Build history of the part. All positions in model axes, mm. Round coordinates to 2 decimals unless told otherwise and drop trailing zeros. Answer in a Markdown table with one row per item.
```python
from build123d import *

# Parameters (mm, degrees)
F1_DEPTH = 3.96875
F2_D     = 6.35
F3_D     = 6.35


with BuildPart() as f1:
    # F0 (on Top) → F1 (new body)
    with BuildSketch(Plane.XY):
        with BuildLine():
            add(Edge.make_bspline(
                [(93.0961013775, 11.8631264067), (73.0208323512, -1.8265877953), (59.8314115865, 0), (7.6732839915, 0)],
                knots=[0, 0, 0, 0, 86.2426315595, 86.2426315595, 86.2426315595, 86.2426315595], degree=3))
            add(Edge.make_bspline(
                [(7.3635370912, 22.8609638917), (45.8569088961, 23.6332072416), (80.4890639518, 17.6334698365), (93.0961013775, 11.8631264067)],
                knots=[0, 0, 0, 0, 86.4350913023, 86.4350913023, 86.4350913023, 86.4350913023], degree=3))
            add(Edge.make_bspline(
                [(-50.7329378175, 20.9600568183), (-28.6348905119, 23.0391732855), (-2.4380154521, 23.6332072416), (7.3635370912, 22.8609638917)],
                knots=[0, 0, 0, 0, 58.1275652726, 58.1275652726, 58.1275652726, 58.1275652726], degree=3))
            add(Edge.make_bspline(
                [(-81.150870805, 19.8313930948), (-72.6527741432, 19.950199886), (-60.8315071405, 19.059149745), (-50.7329378175, 20.9600568183)],
                knots=[0, 0, 0, 0, 30.4388654361, 30.4388654361, 30.4388654361, 30.4388654361], degree=3))
            add(Edge.make_bspline(
                [(-81.150870805, -3.0372931352), (-91.1866208845, 0), (-96.1764965988, 16.4454019242), (-81.150870805, 19.8313930948)],
                knots=[0, 0, 0, 0, 22.8686862301, 22.8686862301, 22.8686862301, 22.8686862301], degree=3))
            add(Edge.make_bspline(
                [(-41.2958105253, -1.8235209079), (-58.2979012822, -1.90700734), (-70.3425093809, 3.5678162715), (-81.150870805, -3.0372931352)],
                knots=[0, 0, 0, 0, 39.8735385051, 39.8735385051, 39.8735385051, 39.8735385051], degree=3))
            add(Edge.make_bspline(
                [(-0.9071079771, -2.6666779982), (-11.7089183609, 7.7004259843), (-20.3979939932, -2.0482919491), (-41.2958105253, -1.8235209079)],
                knots=[0, 0, 0, 0, 40.3975024897, 40.3975024897, 40.3975024897, 40.3975024897], degree=3))
            ThreePointArc((-0.9071079771, -2.6666779982), (2.8162542913, 0.4905240496), (7.6732839915, 0))
        make_face()
    extrude(amount=F1_DEPTH)

    # F2 (through all)
    with Locations(Plane(origin=(0, 0, 0), x_dir=(1, 0, 0), z_dir=(0, 0, -1))):
        with Locations((-49.7787126682, -11.3269922778)):
            Hole(F2_D / 2)

    # F3 (through all)
    with Locations(Plane(origin=(0, 0, 0), x_dir=(1, 0, 0), z_dir=(0, 0, -1))):
        with Locations((-83.2072975638, -10.5645472046), (-17.3172454044, -12.5823580943)):
            Hole(F3_D / 2)


solid = f1.part
```
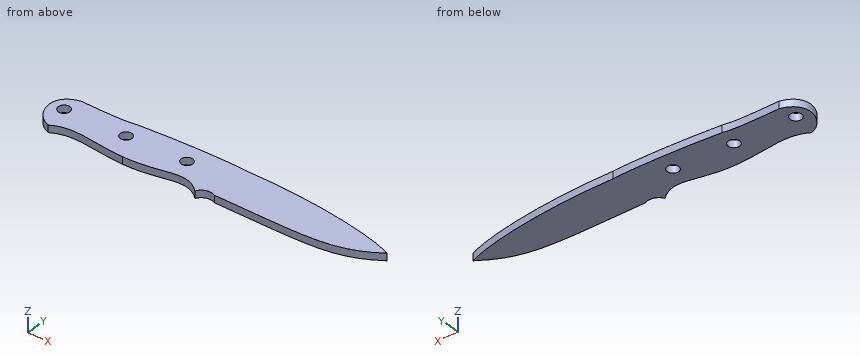
Q1. Drop a flat-ended pin along its axis: P1, Ø4, axis at x = -17.32, y = 12.58, coming from the +Z side. Give the stop position or say it passes through.
A:
| item | result |
|---|---|
| P1 | through |
Q2. Wall check: line 1 (X direction, y = 11.25, z = 3.05); line 2 (X direction, y = 8.5, z = 3); line 3 (X direction, y = 9, z = 2.15). Give the ranges that are in metal, low to high. Write a range as [from, to].
A:
| item | result |
|---|---|
| line 1 | [-90.52, -86.31], [-80.11, -52.95], [-46.6, -20.2], [-14.44, 92.19] |
| line 2 | [-90.58, -85.62], [-80.8, -51.22], [-48.33, 87.76] |
| line 3 | [-90.62, -85.97], [-80.44, -51.94], [-47.62, 88.61] |
Q3. Saw through at A-A on z = 2.6. State how many separate pieces and enclosed holes the cut face has, plus the area to 3 significant figures.
A:
| item | result |
|---|---|
| separate pieces | 1 |
| enclosed holes | 3 |
| area | 3,570 mm² |
